For this review, take the finished solid that the model builds, in its own axes (mm). A direction names the side the tool comes from. Give positions to 0.01 mm unless a question says otherwise; leave off trailing zeros. Order: outer loops, then holes, each group sorted by start corner. A loop starts at its lowest first (then second) coordinate and runs counter-clockwise, first axis right, second up. Notation, with made-up numbers: (19, -3.5) - (41, -3.5) arc R5 cw to (41, 4.5) - close; hole circle Ø6 at (-24, 73). An arc over 180 degrees is marked (long way). One line per item, written item: value.
```python
from build123d import *

# Parameters (mm, degrees)
BOSS_EXTRUDE1_DEPTH      = 37
BOSS_EXTRUDE1_DEPTH_BACK = 45
SKETCH1_R                = 7.4
SKETCH4_W                = 6.2
SKETCH4_H                = 4.7
CUT_EXTRUDE1_DEPTH       = 13
BOSS_EXTRUDE2_DEPTH      = 46
FILLET1_R                = 3


with BuildPart() as part:
    # Sketch1 → Boss-Extrude1 (new, two sides: drawn at the far end of the back side and taken through both)
    with BuildSketch(Plane.XY.offset(-BOSS_EXTRUDE1_DEPTH_BACK)):
        Circle(SKETCH1_R)
    extrude(amount=BOSS_EXTRUDE1_DEPTH + BOSS_EXTRUDE1_DEPTH_BACK)

    # Sketch4 → Cut-Extrude1 (cut)
    with BuildSketch(Plane(origin=(0, 0, -45), x_dir=(-1, 0, 0), z_dir=(0, 0, -1))):
        with Locations((0, 7.4)):
            Rectangle(SKETCH4_W, SKETCH4_H)
    extrude(amount=-CUT_EXTRUDE1_DEPTH, mode=Mode.SUBTRACT)

    # Sketch5 → Boss-Extrude2 (add)
    with BuildSketch(Plane.XY.offset(-23)):
        Polygon((4.419750831, 7.312943041), (-4.123319035, 7.484088019), (-8.543069866, 0.171144977), (-4.419750831, -7.312943041), (4.123319035, -7.484088019), (8.543069866, -0.171144977), align=None)
    extrude(amount=BOSS_EXTRUDE2_DEPTH)

    # Fillet1
    fillet1_edges = [part.edges().sort_by_distance(p)[0] for p in [
        (8.543069866, -0.171144977, 0),
        (4.419750831, 7.312943041, 0),
        (-4.123319035, 7.484088019, 0),
        (-8.543069866, 0.171144977, 0),
        (-4.419750831, -7.312943041, 0),
        (4.123319035, -7.484088019, 0),
    ]]
    fillet(fillet1_edges, radius=FILLET1_R)


solid = part.part
```
(1) Machinability: for faces 1 (the face through (4, 6.5, 23)), 2 (the face through (3.6, -6.7, 23)), 3 (the face through (4, 6.5, -23)), 4 (the face through (-3.8, -6.6, 23)), 5 (the face through (0, 5.05, -39)), which of the approach directions +Z, -Z, +X, -X, +Y, -Y give a long, thin tool a straight path to every point of the face, cutting with its end or side? Answer none if there is none.
Answers below:
face 1: +Z, +X, +Y
face 2: +Z, +X, -Y
face 3: -Z, +X, +Y
face 4: +Z, -X, -Y
face 5: -Z, +Y
(2) Take a section at C-C (z = -28). Write out the cut boundary in (x, y).
Answers below:
outline: circle Ø14.8 at (0, 0)
(3) Take a section at A-A (z = 19). Write out the cut boundary in (x, y), then the cut area to 3 significant figures.
Answers below:
outline: (-7.71, -1.35) - (-5.26, -5.8) arc R3 ccw to (-2.69, -7.35) - (2.39, -7.45) arc R3 ccw to (5.02, -6) - (7.65, -1.65) arc R3 ccw to (7.71, 1.35) - (5.26, 5.8) arc R3 ccw to (2.69, 7.35) - (-2.39, 7.45) arc R3 ccw to (-5.02, 6) - (-7.65, 1.65) arc R3 ccw to start
area: 187 mm^2
(4) Take a section at B-B (y = 0). Write out the cut boundary in (x, z).
Answers below:
outline: (-8.08, -23) - (-7.4, -23) - (-7.4, -45) - (7.4, -45) - (7.4, -23) - (8.08, -23) - (8.08, 23) - (7.4, 23) - (7.4, 37) - (-7.4, 37) - (-7.4, 23) - (-8.08, 23) - close
(5) For P1, Ø6, axis at x = 6.5, z = -19, coming from the -Y side; P2, Ø3, axis at x = 3, z = -3, coming from the +Y side; P3, Ø1.5, axis at x = 4.5, z = -32.5, coming from the +Y side, all flat-tipped, find the tip position at first contact; note any pin that passes through.
Answers below:
P1: stops at y = -7.26
P2: stops at y = 7.37
P3: stops at y = 6.38
(6) Wall thickness on line 1 (X direction, y = 6.5, z = -37); line 2 (Y direction, x = 0.5, z = -7.5); line 3 (X direction, y = 1, z = -32.5): over which ranges is each line inside the solid? List them lowest first. Write a range as from..to.
Answers below:
line 1: x = -3.54..-3.1, 3.1..3.54
line 2: y = -7.41..7.39
line 3: x = -7.33..7.33
(7) Draft analysis for pull direction X (two halves, no side actions). For faces 6 (the face through (-3.8, -6.6, -23)), 7 (the face through (0, 6, -32)), 8 (the face through (-6.5, -3.54, -0.32)), state which applies: pulls with the +X half, pulls with the -X half, needs draft (parallel to the pull), parting line crosses it, or undercut.
Answers below:
face 6: needs draft
face 7: undercut
face 8: pulls with the -X half
